from build123d import *

# Parameters (mm, degrees)
SKETCH_1_W          = 15
SKETCH_1_H          = 5
SKETCH_1_R          = 2.1
SKETCH_1_R_2        = 1
EXTRUDE_1_DEPTH     = 3
EXTRUDE_2_DEPTH     = 2.5
SKETCH_1_3_R        = 1
CUT_EXTRUDE_1_DEPTH = 6
SKETCH_1_4_R        = 2.1
CUT_EXTRUDE_2_DEPTH = 1.4
SKETCH_4_W          = 2.075
SKETCH_4_H          = 2
SKETCH_5_R          = 2.075
CUT_EXTRUDE_3_DEPTH = 1


with BuildPart() as part:
    # Sketch 1 → Extrude 1 (new body)
    with BuildSketch(Plane(origin=(0, 0, 0), x_dir=(1, 0, 0), z_dir=(0, 1, 0))):
        Rectangle(SKETCH_1_W, SKETCH_1_H)
        with Locations((-5, 0)):
            Circle(SKETCH_1_R, mode=Mode.SUBTRACT)
        with Locations((5, 0)):
            Circle(SKETCH_1_R, mode=Mode.SUBTRACT)
        Circle(SKETCH_1_R_2, mode=Mode.SUBTRACT)
        with Locations((-5, 0)):
            Circle(SKETCH_1_R)
        with Locations((5, 0)):
            Circle(SKETCH_1_R)
        Circle(SKETCH_1_R_2)
    extrude(amount=EXTRUDE_1_DEPTH)

    # Sketch 2 → Extrude 2 (add, symmetric)
    with BuildSketch(Plane.XY):
        Polygon((-2.5, 3), (-6.5, 5), (-7.5, 3), align=None)
        Polygon((2.5, 3), (-1.5, 5), (-2.5, 3), align=None)
        Polygon((3.5, 5), (2.5, 3), (7.5, 3), align=None)
    extrude(amount=EXTRUDE_2_DEPTH, both=True)

    # Sketch 1_3 → Cut-Extrude 1 (cut, through all)
    with BuildSketch(Plane(origin=(0, 0, 0), x_dir=(1, 0, 0), z_dir=(0, 1, 0))):
        Circle(SKETCH_1_3_R)
    extrude(amount=CUT_EXTRUDE_1_DEPTH, mode=Mode.SUBTRACT)

    # Sketch 1_4 → Cut-Extrude 2 (cut)
    with BuildSketch(Plane(origin=(0, 0, 0), x_dir=(1, 0, 0), z_dir=(0, 1, 0))):
        with Locations((-5, 0)):
            Circle(SKETCH_1_4_R)
        with Locations((5, 0)):
            Circle(SKETCH_1_4_R)
    extrude(amount=CUT_EXTRUDE_2_DEPTH, mode=Mode.SUBTRACT)

    # Sketch 4 → Cut-Revolve 1 (revolve, cut)
    with BuildSketch(Plane.XY):
        Polygon((2.075, 3), (0, 3), (0, 1.8), (1.075, 1.8), align=None)
        with Locations((1.0375, 4)):
            Rectangle(SKETCH_4_W, SKETCH_4_H)
    revolve(axis=Axis((0, 0, 0), (0, 1, 0)), mode=Mode.SUBTRACT)

    # Sketch 5 → Cut-Extrude 3 (cut)
    with BuildSketch(Plane.XZ):
        Circle(SKETCH_5_R)
    extrude(amount=-CUT_EXTRUDE_3_DEPTH, mode=Mode.SUBTRACT)


solid = part.part
Geometry: final body of the model. Coordinates: model frame, mm. A direction names the side the tool comes from. Give positions to 0.01 mm unless a question says otherwise; leave off trailing zeros. Write each loop counter-clockwise with the first axis right and the second up, starting at its lowest first coordinate (ties: lowest second). Pieces come first, ordered by that corner, then holes. Notation, with made-up numbers: M 58,-26 L 103,-26 A22 ccw 103,-11 Z; hole C 6.25,87 d8. An arc over 180 degrees is marked long. Answer in a Markdown table with one row per item. Add a question column.
(1) Reachability of faces 1 (the cylindrical face through (-2.073, 3.347, -0.091)), 2 (the flat face through (-2, 4, 1)), 3 (the cylindrical face through (7.003, 0.69, -0.631)) from +Z, -Z, +X, -X, +Y, -Y: full face, straight path, thin tool, end or side. Return the list, or none.
(2) First-contact query: pin 1 (1 mm diameter, centred on x = 0.5, z = 1, fed in from -Y); pin 2 (2.5 mm diameter, centred on x = 0.5, z = -0.5, fed in from +Y). Flat tips, straight axial feed; report the tip coordinate or a pass-through.
(3) Section A-A on x = 0. Return loops of the section in (y, z) (3 decimals).
(4) Ray query, line 1 (Z direction, x = 0, y = 0.6) (3 decimals); line 2 (X direction, y = 3.4, z = -2.15); line 3 (X direction, y = 1.15, z = 1.6). Return the intervals inside material, ascending.
(5) Section B-B on y = 0.75. Return loops of the section in (x, z) (3 decimals), and give its area (3 significant figures).
(6) Section C-C on x = 5. Return loops of the section in (y, z), and give its area (3 significant figures).
Result set:
| question | item | result |
|---|---|---|
| 1 | face 1 | +Y |
| 1 | face 2 | +Z, -Z, +Y |
| 1 | face 3 | -Y |
| 2 | pin 1 | stops at y = 1 |
| 2 | pin 2 | stops at y = 2.86 |
| 3 | outline | M 0,-2.5 L 4.25,-2.5 L 4.25,-2.075 L 3,-2.075 L 1.8,-1.075 L 1.8,-1 L 1,-1 L 1,-2.075 L 0,-2.075 Z; M 0,2.075 L 1,2.075 L 1,1 L 1.8,1 L 1.8,1.075 L 3,2.075 L 4.25,2.075 L 4.25,2.5 L 0,2.5 Z |
| 4 | line 1 | z = -2.5 to -2.075, 2.075 to 2.5 |
| 4 | line 2 | x = -7.3 to -3.3, -2.3 to 1.7, 2.7 to 6.7 |
| 4 | line 3 | x = -7.5 to -6.36, -3.64 to 3.64, 6.36 to 7.5 |
| 5 | outline | M -7.5,-2.5 L 7.5,-2.5 L 7.5,2.5 L -7.5,2.5 Z; hole C -5,0 d4.2; hole C 0,0 d4.15; hole C 5,0 d4.2 |
| 5 | area | 33.8 mm^2 |
| 6 | outline | M 0,-2.5 L 4.25,-2.5 L 4.25,2.5 L 0,2.5 L 0,2.1 L 1.4,2.1 L 1.4,-2.1 L 0,-2.1 Z |
| 6 | area | 15.4 mm^2 |
